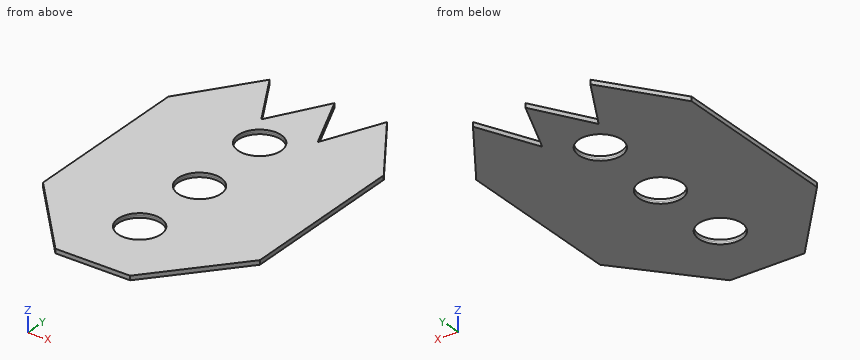
```python
from build123d import *

# Parameters (mm, degrees)
F0_W     = 100
F0_H     = 150
F1_DEPTH = 1
F2_R     = 10
F3_DEPTH = 25
F5_DEPTH = 25
F8_DEPTH = 25
F7_R     = 10
F9_DEPTH = 1


with BuildPart() as f1:
    # F0 (on Top) → F1 (new body)
    with BuildSketch(Plane.XY):
        with Locations((-8.1639520824, 60.1602055132)):
            Rectangle(F0_W, F0_H)
    extrude(amount=F1_DEPTH)

    # F2 (on face) → F3 (cut)
    with BuildSketch(Plane.XY.offset(1)):
        with Locations((-10.0705353543, 94.5251360536)):
            Circle(F2_R)
        with Locations((-9.4941006973, 17.237842083)):
            Circle(F2_R)
        with Locations((-9.2731751502, 55.1192685962)):
            Circle(F2_R)
    extrude(amount=-F3_DEPTH, mode=Mode.SUBTRACT)

    # F4 (on face) → F5 (cut)
    with BuildSketch(Plane.XY.offset(1)):
        Polygon((41.8360479176, 23.1922029477), (9.3773484498, -14.8397944868), (41.8360479176, -14.8397944868), align=None)
        Polygon((-25.1544182483, -14.8397944868), (-58.1639520824, 22.7151076707), (-58.1639520824, -14.8397944868), align=None)
    extrude(amount=-F5_DEPTH, mode=Mode.SUBTRACT)

    # F6 (on face) → F8 (cut)
    with BuildSketch(Plane.XY.offset(1)):
        Polygon((-4.9593081612, 135.1602055132), (-34.9667105038, 135.1602055132), (-19.9630093325, 109.1815806235), align=None)
        Polygon((19.3310942209, 135.1602055132), (-4.9593081612, 135.1602055132), (7.1858930298, 107.7285798226), align=None)
        Polygon((41.8360479176, 135.1602055132), (19.3310942209, 135.1602055132), (41.8360479176, 102.0916848462), align=None)
        Polygon((-58.1639520824, 135.1602055132), (-58.1639520824, 102.5735827495), (-34.9667105038, 135.1602055132), align=None)
    extrude(amount=-F8_DEPTH, mode=Mode.SUBTRACT)

    # F7 (on face) → F9 (join)
    with BuildSketch(Plane.XY.offset(1)):
        Polygon((-19.9630093325, 109.1815806235), (-34.9667105038, 135.1602055132), (-58.1639520824, 102.5735827495), (-58.1639520824, 22.7151076707), (-25.1544182483, -14.8397944868), (9.3773484498, -14.8397944868), (41.8360479176, 23.1922029477), (41.8360479176, 102.0916848462), (19.3310942209, 135.1602055132), (7.1858930298, 107.7285798226), (-4.9593081612, 135.1602055132), align=None)
        with Locations((-9.4941006973, 17.237842083)):
            Circle(F7_R, mode=Mode.SUBTRACT)
        with Locations((-9.2731751502, 55.1192685962)):
            Circle(F7_R, mode=Mode.SUBTRACT)
        with Locations((-10.0705353543, 94.5251360536)):
            Circle(F7_R, mode=Mode.SUBTRACT)
    extrude(amount=F9_DEPTH)


solid = f1.part
```
Geometry check sheet. Reference: the model listing, model coordinates, mm. Coordinates: 2 decimals unless noted, no trailing zeros. Write each loop counter-clockwise with the first axis right and the second up, starting at its lowest first coordinate (ties: lowest second). Pieces come first, ordered by that corner, then holes. Notation, with made-up numbers: M -17,3.25 L 33,3.25 A10 cw 33,16.25 Z; hole C -5.75,2.25 d10. An arc over 180 degrees is marked long. Use one line per item in the form item = value. Start each with the question number.
1) Section check C-C on x = -6.5. Enter the section's corners in (y, z), and give its area (3 significant figures).
2) Section check A-A on y = 118. Enter the section's corners in (x, z), and give its area (3 significant figures).
3) Thickness scan on probe 1 along Y at (x, z) = (-13, 1.1); probe 2 along X at (y, z) = (94.5, 0.7); probe 3 along X at (y, z) = (18, 1.3). Record the ranges inside material, lowest first. Write a range as from..to.
4) Go/stop test with a flat-tipped pin: pin 1 Ø18 at (x, y) = (-10.07, 94.53) entering from -Z. Record where the tip stops, or that it passes through.
5) Section check B-B on z = 1.65. Enter the section's corners in (x, y).
6) Section check D-D on x = 12. Enter the section's corners in (y, z), and give its area (3 significant figures).
Responses:
q1.outline = M -14.84,0 L 7.7,0 L 7.7,2 L -14.84,2 Z; M 26.78,0 L 45.51,0 L 45.51,2 L 26.78,2 Z; M 64.73,0 L 85.18,0 L 85.18,2 L 64.73,2 Z; M 103.87,0 L 132.49,0 L 132.49,2 L 103.87,2 Z
q1.area = 181 mm2
q2.outline = M -47.18,0 L -25.06,0 L -25.06,2 L -47.18,2 Z; M -14.87,0 L 2.64,0 L 2.64,2 L -14.87,2 Z; M 11.73,0 L 31.01,0 L 31.01,2 L 11.73,2 Z
q2.area = 118 mm2
q3.probe_1 = -14.84..7.87, 26.6..45.84, 64.4..84.96, 104.09..121.24
q3.probe_2 = -58.16..-20.07, -0.07..41.84
q3.probe_3 = -54.02..-19.47, 0.48..37.4
q4.pin_1 = through
q5.outline = M -58.16,22.72 L -25.15,-14.84 L 9.38,-14.84 L 41.84,23.19 L 41.84,102.09 L 19.33,135.16 L 7.19,107.73 L -4.96,135.16 L -19.96,109.18 L -34.97,135.16 L -58.16,102.57 Z; hole C -10.07,94.53 d20; hole C -9.49,17.24 d20; hole C -9.27,55.12 d20
q6.outline = M -11.77,0 L 118.6,0 L 118.6,2 L -11.77,2 Z
q6.area = 261 mm2
